For this review, take the finished solid that the model builds, in its own axes (mm). A direction names the side the tool comes from. Coordinates: 2 decimals unless noted, no trailing zeros. Loops run counter-clockwise (first coordinate to the right, second up) from the corner with the lowest first, then second, coordinate; pieces in that order, holes last. Notation, with made-up numbers: (20, 13) - (77, 13) arc R15 ccw to (77, 26) - close; hole circle Ø1 at (30, 87.5). An arc over 180 degrees is marked (long way). Answer as a JSON object with one key per item and string values. Group by question number.
Item 1: Clearance check with flat-ended pins moving along their axes: pin 1 (3.5 mm diameter, centred on x = 21.33, z = 0, fed in from +Y); pin 2 (4.5 mm diameter, centred on x = -0.37, z = 0, fed in from +Y); pin 3 (1 mm diameter, centred on y = 2.5, z = 1.5, fed in from +X). State where each tip first meets the part, or that it passes through.
Item 2: We need section D-D (x = -10.5). Give the boundary of the cut face in (y, z).
Item 3: We need section C-C (y = 1.3). Give the boundary of the cut face in (x, z), then the cut area to 3 significant figures.
Item 4: Mouldability with a two-part tool opening along X and no side actions: class faces 1 (the cylindrical face through (35.22, 1.48, -0.07)), 2 (the cylindrical face through (19.374, 1.479, -0.434)), 3 (the flat face through (-0.5, 0, -2.3)) as released by +X, released by -X, zero draft, split by the parting line, or undercut.
Item 5: We need section B-B (x = 6). Give the boundary of the cut face in (y, z).
Item 6: Tool access review of faces 4 (the cylindrical face through (16.078, 1.479, -0.26)), 5 (the flat face through (2, 1, 3.087)), 6 (the flat face through (2, 1, -3.087)): name each direction out of +Z, -Z, +X, -X, +Y, -Y from which nothing blocks a thin tool from reaching the whole face with its end or side.
Item 7: To check wall thickness, follow line 1 (Z direction, x = 16.5, y = 0.3); line 2 (Z direction, x = 8, y = 1.9); line 3 (Z direction, x = -30, y = 2.65). State the ranges of each line that lie inside material, in increasing order.
Item 8: We need section A-A (z = 0). Give the boundary of the cut face in (x, y), then the cut area to 3 significant figures.
from build123d import *

# Parameters (mm, degrees)
SKETCH2_R           = 2
BOSS_EXTRUDE2_DEPTH = 3
SKETCH6_R           = 5
BOSS_EXTRUDE5_DEPTH = 3
SKETCH8_R           = 2
CUT_EXTRUDE3_DEPTH  = 10


with BuildPart() as part:
    # Sketch2 → Boss-Extrude2 (new body)
    with BuildSketch(Plane(origin=(0, 0, 0), x_dir=(1, 0, 0), z_dir=(0, 1, 0))):
        with BuildLine():
            Line((-32.1334036, 3.086573492), (32.1334036, 3.086573492))
            ThreePointArc((32.1334036, 3.086573492), (35.219977092, 0), (32.1334036, -3.086573492))
            Line((32.1334036, -3.086573492), (-32.1334036, -3.086573492))
            Line((-32.1334036, -3.086573492), (-32.1334036, 3.086573492))
        make_face()
        with Locations(Location((28.558761332, 0, 0), (0, 0, 270))):
            Circle(SKETCH2_R, mode=Mode.SUBTRACT)
        with Locations(Location((21.326683463, 0, 0), (0, 0, 270))):
            Circle(SKETCH2_R, mode=Mode.SUBTRACT)
        with Locations(Location((14.094605594, 0, 0), (0, 0, 270))):
            Circle(SKETCH2_R, mode=Mode.SUBTRACT)
        with Locations(Location((6.862527725, 0, 0), (0, 0, 270))):
            Circle(SKETCH2_R, mode=Mode.SUBTRACT)
        with Locations(Location((-0.369550144, 0, 0), (0, 0, 270))):
            Circle(SKETCH2_R, mode=Mode.SUBTRACT)
    extrude(amount=BOSS_EXTRUDE2_DEPTH)

    # Sketch6 → Boss-Extrude5 (add)
    with BuildSketch(Plane(origin=(0, 3, 0), x_dir=(1, 0, 0), z_dir=(0, 1, 0))):
        with Locations((-32.1334036, 0)):
            Circle(SKETCH6_R)
    extrude(amount=-BOSS_EXTRUDE5_DEPTH)

    # Sketch8 → Cut-Extrude3 (cut)
    with BuildSketch(Plane(origin=(0, 3, 0), x_dir=(1, 0, 0), z_dir=(0, 1, 0))):
        with Locations(Location((-32.1334036, 0, 0), (0, 0, 270))):
            Circle(SKETCH8_R)
    extrude(amount=-CUT_EXTRUDE3_DEPTH, mode=Mode.SUBTRACT)


solid = part.part
Check sheet entries:
{
 "1": {"pin 1": "passes through", "pin 2": "stops at y = 3", "pin 3": "stops at x = 35.05"},
 "2": {"outline": "(0, -3.09) - (3, -3.09) - (3, 3.09) - (0, 3.09) - close"},
 "3": {"outline": "(-28.2, -3.09) - (32.13, -3.09) arc R3.09 ccw to (32.13, 3.09) - (-28.2, 3.09) arc R5 ccw (long way) to start; hole circle Ø4 at (-32.13, 0); hole circle Ø4 at (-0.37, 0); hole circle Ø4 at (6.86, 0); hole circle Ø4 at (14.09, 0); hole circle Ø4 at (21.33, 0); hole circle Ø4 at (28.56, 0)", "area": "386 mm2"},
 "4": {"face 1": "released by +X", "face 2": "undercut", "face 3": "zero draft"},
 "5": {"outline": "(0, -3.09) - (3, -3.09) - (3, -1.8) - (0, -1.8) - close; (0, 1.8) - (3, 1.8) - (3, 3.09) - (0, 3.09) - close"},
 "6": {"face 4": "+Y, -Y", "face 5": "+Z, +X, +Y, -Y", "face 6": "-Z, +X, +Y, -Y"},
 "7": {"line 1": "z = -3.09 to 3.09", "line 2": "z = -3.09 to -1.65, 1.65 to 3.09", "line 3": "z = -4.52 to 4.52"},
 "8": {"outline": "(-37.13, 0) - (-34.13, 0) - (-34.13, 3) - (-37.13, 3) - close; (-30.13, 0) - (-2.37, 0) - (-2.37, 3) - (-30.13, 3) - close; (1.63, 0) - (4.86, 0) - (4.86, 3) - (1.63, 3) - close; (8.86, 0) - (12.09, 0) - (12.09, 3) - (8.86, 3) - close; (16.09, 0) - (19.33, 0) - (19.33, 3) - (16.09, 3) - close; (23.33, 0) - (26.56, 0) - (26.56, 3) - (23.33, 3) - close; (30.56, 0) - (35.22, 0) - (35.22, 3) - (30.56, 3) - close", "area": "145 mm2"}
}
